from build123d import *
from build123d.topology import SkipClean

# Parameters (mm, degrees)
SKIZZE1_R                       = 12
SKIZZE1_R_2                     = 1.5
AUFSATZ_LINEAR_AUSTRAGEN1_DEPTH = 18
AUFSATZ_LINEAR_START            = 1
SKIZZE4_R                       = 15
SKIZZE4_R_2                     = 1.5
AUFSATZ_LINEAR_AUSTRAGEN2_DEPTH = 1
SKIZZE2_R                       = 2.9
SCHNITT_LINEAR_AUSTRAGEN4_DEPTH = 14
SCHNITT_LINEAR_AUSTRAGEN5_DEPTH = 23
SKIZZE9_R                       = 2.5
SCHNITT_LINEAR_AUSTRAGEN7_DEPTH = 5


with BuildPart() as part:
    # Skizze1 → Aufsatz-Linear austragen1 (new body)
    with BuildSketch(Plane.XY):
        Circle(SKIZZE1_R)
        with Locations((9, 0)):
            Circle(SKIZZE1_R_2, mode=Mode.SUBTRACT)
        with Locations((0, -9)):
            Circle(SKIZZE1_R_2, mode=Mode.SUBTRACT)
        with Locations((-9, 0)):
            Circle(SKIZZE1_R_2, mode=Mode.SUBTRACT)
        with Locations((0, 9)):
            Circle(SKIZZE1_R_2, mode=Mode.SUBTRACT)
    extrude(amount=AUFSATZ_LINEAR_AUSTRAGEN1_DEPTH)

    # Skizze4 → Aufsatz-Linear austragen2 (add)
    with SkipClean():  # the faces are left unmerged after this step: merging them gives an invalid solid
        with BuildSketch(Plane(origin=(0, 0, 0), x_dir=(-1, 0, 0), z_dir=(0, 0, -1)).offset(AUFSATZ_LINEAR_START)):
            Circle(SKIZZE4_R)
            with Locations((0, 9)):
                Circle(SKIZZE4_R_2, mode=Mode.SUBTRACT)
            with Locations((9, 0)):
                Circle(SKIZZE4_R_2, mode=Mode.SUBTRACT)
            with Locations((0, -9)):
                Circle(SKIZZE4_R_2, mode=Mode.SUBTRACT)
            with Locations((-9, 0)):
                Circle(SKIZZE4_R_2, mode=Mode.SUBTRACT)
        extrude(amount=-AUFSATZ_LINEAR_AUSTRAGEN2_DEPTH)

    # Skizze2 → Schnitt-Linear austragen4 (cut)
    with BuildSketch(Plane.XY.offset(18)):
        with Locations((0, 9)):
            Circle(SKIZZE2_R)
        with Locations((9, 0)):
            Circle(SKIZZE2_R)
        with Locations((0, -9)):
            Circle(SKIZZE2_R)
        with Locations((-9, 0)):
            Circle(SKIZZE2_R)
    extrude(amount=-SCHNITT_LINEAR_AUSTRAGEN4_DEPTH, mode=Mode.SUBTRACT)

    # Skizze6 → Schnitt-Linear austragen5 (cut)
    with BuildSketch(Plane.XY.offset(18)):
        with BuildLine():
            Line((1.5, 2), (-1.5, 2))
            ThreePointArc((-1.5, 2), (-1.118033989, -2.236067977), (2.5, 0))
            ThreePointArc((2.5, 0), (2.236067977, 1.118033989), (1.5, 2))
        make_face()
    extrude(amount=-SCHNITT_LINEAR_AUSTRAGEN5_DEPTH, mode=Mode.SUBTRACT)

    # Skizze9 → Schnitt-Linear austragen7 (cut)
    with BuildSketch(Plane.XY.offset(18)):
        Circle(SKIZZE9_R)
    extrude(amount=-SCHNITT_LINEAR_AUSTRAGEN7_DEPTH, mode=Mode.SUBTRACT)


solid = part.part
Input: part model. Units: mm. Frame: model coordinates. A direction names the side the tool comes from. Give positions to 0.01 mm unless a question says otherwise; leave off trailing zeros. Order: outer loops, then holes, each group sorted by start corner. A loop starts at its lowest first (then second) coordinate and runs counter-clockwise, first axis right, second up. Notation, with made-up numbers: (41, -36.5) - (69, -36.5) arc R28 ccw to (69, -9.5) - close; hole circle Ø11 at (5, 82.25). An arc over 180 degrees is marked (long way). Answer as a JSON object with one key per item and string values. Group by question number.
Q1. Line query: probe 1 along Y at (x, z) = (1, 14.25); probe 2 along Y at (x, z) = (9, -0.5); probe 3 along Z at (x, y) = (-10, 1.25). Output: solid intervals per line, ascending.
Q2. First-contact query: pin 1 Ø1.5 at (x, z) = (8.5, 12) entering from +Y; pin 2 Ø1.5 at (y, z) = (-1, 12.5) entering from -X; pin 3 Ø4 at (y, z) = (11, 8.5) entering from -X. Flat tips, straight axial feed; report the tip coordinate or a pass-through.
Q3. Cut plane D-D, the plane x = -9.5. Output: boundary loops of the cut face in (y, z).
Q4. Cut plane B-B, the plane y = 0.75. Output: boundary loops of the cut face in (x, z), then the cut area to 3 significant figures.
Q5. Set-up query: faces 4 (the face through (-3, 0, -1)), 5 (the face through (-11.301, -1.765, 11.098)). Return all of +Z, -Z, +X, -X, +Y, -Y with unobstructed straight access to the full face (end or side cutting, diameter ignored); none if empty.
Q6. Cut plane A-A, the plane z = 11.75. Output: boundary loops of the cut face in (x, y).
Q7. Mould query, pull axis Y, two halves, no side actions, for faces 1 (the face through (7, 10, 0)), 2 (the face through (0, 2, 6)), 3 (the face through (14.985, 0.66, -0.507)). Classes: pulls with the +Y half, pulls with the -Y half, needs draft (parallel to the pull), parting line crosses it, or undercut.
Results:
{
 "1": {"probe 1": "-11.96 to -11.72, -6.28 to -2.29, 2.29 to 6.28, 11.72 to 11.96", "probe 2": "-12 to -1.5, 1.5 to 12", "probe 3": "-1 to 4"},
 "2": {"pin 1": "y = 9.16", "pin 2": "x = -12", "pin 3": "x = -7.94"},
 "3": {"outline": "(-11.61, -1) - (-1.41, -1) - (-1.41, 4) - (-2.86, 4) - (-2.86, 18) - (-7.33, 18) - (-7.33, 0) - (-11.61, 0) - close; (1.41, -1) - (11.61, -1) - (11.61, 0) - (7.33, 0) - (7.33, 18) - (2.86, 18) - (2.86, 4) - (1.41, 4) - close"},
 "4": {"outline": "(-14.98, -1) - (-10.3, -1) - (-10.3, 4) - (-11.8, 4) - (-11.8, 18) - (-11.98, 18) - (-11.98, 0) - (-14.98, 0) - close; (-7.7, -1) - (-2.38, -1) - (-2.38, 18) - (-6.2, 18) - (-6.2, 4) - (-7.7, 4) - close; (2.38, -1) - (7.7, -1) - (7.7, 4) - (6.2, 4) - (6.2, 18) - (2.38, 18) - close; (10.3, -1) - (14.98, -1) - (14.98, 0) - (11.98, 0) - (11.98, 18) - (11.8, 18) - (11.8, 4) - (10.3, 4) - close", "area": "188 mm^2"},
 "5": {"face 4": "-Z, +X, -X, +Y, -Y", "face 5": "+Z"},
 "6": {"outline": "circle Ø24 at (0, 0); hole circle Ø5.8 at (-9, 0); hole circle Ø5.8 at (0, -9); hole circle Ø5.8 at (0, 9); hole (-1.5, 2) arc R2.5 ccw (long way) to (1.5, 2) - close; hole circle Ø5.8 at (9, 0)"},
 "7": {"face 1": "needs draft", "face 2": "undercut", "face 3": "parting line crosses it"}
}
